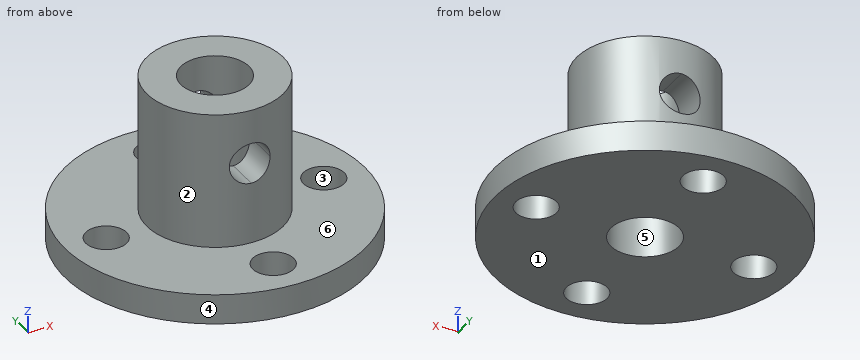
from build123d import *

# Parameters (mm, degrees)
SKETCH_1_R               = 11
SKETCH_1_R_2             = 1.5
EXTRUDE_1_DEPTH          = 2.2
SKETCH_2_R               = 5
EXTRUDE_2_DEPTH          = 10
SKETCH_3_R               = 2.5
CUT_EXTRUDE_1_DEPTH      = 20.769673745
CUT_EXTRUDE_2_DEPTH      = 20.769673745
CUT_EXTRUDE_2_DEPTH_BACK = 20.769673745


with BuildPart() as part:
    # 草图1 → 凸台-拉伸1 (new body)
    with BuildSketch(Plane.XY):
        Circle(SKETCH_1_R)
        with Locations((0, 8)):
            Circle(SKETCH_1_R_2, mode=Mode.SUBTRACT)
        with Locations((8, 0)):
            Circle(SKETCH_1_R_2, mode=Mode.SUBTRACT)
        with Locations((0, -8)):
            Circle(SKETCH_1_R_2, mode=Mode.SUBTRACT)
        with Locations((-8, 0)):
            Circle(SKETCH_1_R_2, mode=Mode.SUBTRACT)
    extrude(amount=EXTRUDE_1_DEPTH)

    # 草图2 → 凸台-拉伸2 (add)
    with BuildSketch(Plane.XY.offset(2.2)):
        Circle(SKETCH_2_R)
    extrude(amount=EXTRUDE_2_DEPTH)

    # 草图3 → 切除-拉伸1 (cut, through all)
    with BuildSketch(Plane.XY.offset(12.2)):
        Circle(SKETCH_3_R)
    extrude(amount=-CUT_EXTRUDE_1_DEPTH, mode=Mode.SUBTRACT)

    # 草图4 → 切除-拉伸2 (cut, two sides: drawn at the far end of the back side and taken through both)
    with BuildSketch(Plane(origin=(0, 0, 0), x_dir=(1, 0, 0), z_dir=(0, 1, 0)).offset(-CUT_EXTRUDE_2_DEPTH_BACK)):
        with BuildLine():
            ThreePointArc((1.5, -8.2), (1.060660172, -7.139339828), (0, -6.7))
            Line((0, -6.7), (0, -9.7))
            ThreePointArc((0, -9.7), (1.060660172, -9.260660172), (1.5, -8.2))
        make_face()
        with BuildLine():
            Line((0, -9.7), (0, -6.7))
            ThreePointArc((0, -6.7), (-1.5, -8.2), (0, -9.7))
        make_face()
    extrude(amount=CUT_EXTRUDE_2_DEPTH + CUT_EXTRUDE_2_DEPTH_BACK, mode=Mode.SUBTRACT)


solid = part.part
Design review of the part built by this model. Coordinates are the model's own, in mm. Face numbers are marked on the shaded views. A direction names the side the tool comes from. Round coordinates to 2 decimals unless told otherwise and drop trailing zeros. Loops run counter-clockwise (first coordinate to the right, second up) from the corner with the lowest first, then second, coordinate; pieces in that order, holes last. Notation, with made-up numbers: (63, 30.5) - (79, 30.5) arc R13 cw to (79, 43.5) - close; hole circle Ø4 at (47, 10). An arc over 180 degrees is marked (long way). One line per item, written item: value. Start each with the question number.
1) Draft analysis for pull direction X (two halves, no side actions). For the marked faces 3, 4, 5 and 6, state which applies: +X half, -X half, draft (parallel to the pull), parting line (faces both ways), or undercut.
2) Consider section B-B on z = 1.75. Give the boundary of the cut face in (x, y).
3) Consider section C-C on x = 8. Give the boundary of the cut face in (y, z).
4) Consider section A-A on y = 0. Give the boundary of the cut face in (x, z).
5) Insertion check: pin 1 Ø2 at (x, z) = (-3.5, 1.5) entering from +Y; pin 2 Ø3.5 at (x, y) = (0, 8) entering from -Z; pin 3 Ø6 at (x, y) = (-5.5, 7.5) entering from +Z. Each pin has a flat end and moves straight along its axis. Give the tip position at first contact, or say it passes through.
6) For the marked faces 1 and 2, list the 3-axis set-ups (+Z, -Z, +X, -X, +Y, -Y) from which the entire face can be reached by the end or side of a thin tool; tool diameter is ignored.
7) To check wall thickness, follow L1, parallel to Y at x = 0, z = 0.75; L2, parallel to Y at x = 0, z = 11.75; L3, parallel to Z at x = 5.25, y = -8. State the ranges of each line that lie inside material, in increasing order. Write a range as from..to.
Reported:
1. face 3: undercut
1. face 4: parting line
1. face 5: undercut
1. face 6: draft
2. outline: circle Ø22 at (0, 0); hole circle Ø3 at (-8, 0); hole circle Ø5 at (0, 0); hole circle Ø3 at (0, -8); hole circle Ø3 at (0, 8); hole circle Ø3 at (8, 0)
3. outline: (-7.55, 0) - (-1.5, 0) - (-1.5, 2.2) - (-7.55, 2.2) - close; (1.5, 0) - (7.55, 0) - (7.55, 2.2) - (1.5, 2.2) - close
4. outline: (-11, 0) - (-9.5, 0) - (-9.5, 2.2) - (-11, 2.2) - close; (-6.5, 0) - (-2.5, 0) - (-2.5, 12.2) - (-5, 12.2) - (-5, 2.2) - (-6.5, 2.2) - close; (2.5, 0) - (6.5, 0) - (6.5, 2.2) - (5, 2.2) - (5, 12.2) - (2.5, 12.2) - close; (9.5, 0) - (11, 0) - (11, 2.2) - (9.5, 2.2) - close
5. pin 1: stops at y = 10.71
5. pin 2: stops at z = 0
5. pin 3: stops at z = 2.2
6. face 1: -Z, +X, -X, +Y, -Y
6. face 2: +Z
7. L1: y = -11..-9.5, -6.5..-2.5, 2.5..6.5, 9.5..11
7. L2: y = -5..-2.5, 2.5..5
7. L3: z = 0..2.2
